from build123d import *

# Parameters (mm, degrees)
EXTRUDE_6_DEPTH           = 20
SKETCH_6_W                = 17.85
SKETCH_6_H                = 4
EXTRUDE_7_DEPTH           = 8
SKETCH_7_W                = 17.85
SKETCH_7_H                = 4
EXTRUDE_8_DEPTH           = 8
SKETCH_10_R               = 1.975
CUT_EXTRUDE_5_DEPTH       = 23.9
SKETCH_9_W                = 11
SKETCH_9_H                = 10.2
CUT_EXTRUDE_7_DEPTH       = 22
SKETCH_12_R               = 3.5
CUT_EXTRUDE_8_DEPTH       = 2.9
CUT_EXTRUDE_9_DEPTH       = 3.2
EXTRUDE_11_DEPTH          = 4
EXTRUDE_START             = -20
EXTRUDE_12_DEPTH          = 20
CUT_EXTRUDE_12_DEPTH      = 10
SKETCH_20_W               = 6
SKETCH_20_H               = 4
CUT_EXTRUDE_13_DEPTH      = 10
REVOLVE_1_ANGLE           = 180
EXTRUDE_13_DEPTH          = 30
SKETCH_38_W               = 28
SKETCH_38_H               = 8
EXTRUDE_14_DEPTH          = 34
SKETCH_37_W               = 8.80839151
SKETCH_37_H               = 35.661760673
CUT_EXTRUDE_15_DEPTH      = 22.758116413
CUT_EXTRUDE_15_DEPTH_BACK = 58.758116413
SKETCH_40_W               = 21.302771057
SKETCH_40_H               = 34
CUT_EXTRUDE_16_DEPTH      = 7
CUT_EXTRUDE_16_DEPTH_BACK = 40.8500001
SKETCH_42_W               = 6
SKETCH_42_H               = 6
CUT_EXTRUDE_17_DEPTH      = 29.0000001
FILLET_1_R                = 5
FILLET_2_R                = 2


with BuildPart() as part:
    # 스케치1 → 보스-돌출6 (new body)
    with BuildSketch(Plane.XY):
        Polygon((-42.18773019, 15.20361991), (-19.28773019, 15.20361991), (-19.28773019, -6.79638009), (3.66226981, -6.79638009), (3.66226981, -77.79638009), (-42.18773019, -77.79638009), (-42.18773019, -73.79638009), (-16.33773019, -73.79638009), (-16.33773019, -26.79638009), (-42.18773019, -26.79638009), align=None)
    extrude(amount=EXTRUDE_6_DEPTH)

    # 스케치6 → 보스-돌출7 (add)
    with BuildSketch(Plane.XY.offset(20)):
        with Locations((-33.26273019, -75.79638009)):
            Rectangle(SKETCH_6_W, SKETCH_6_H)
    extrude(amount=EXTRUDE_7_DEPTH)

    # 스케치7 → 보스-돌출8 (add)
    with BuildSketch(Plane(origin=(0, 0, 0), x_dir=(-1, 0, 0), z_dir=(0, 0, -1))):
        with Locations((33.26273019, -75.79638009)):
            Rectangle(SKETCH_7_W, SKETCH_7_H)
    extrude(amount=EXTRUDE_8_DEPTH)

    # 스케치10 → 컷-돌출5 (cut, through all)
    with BuildSketch(Plane(origin=(-19.28773019, 0, 0), x_dir=(0, 0, -1), z_dir=(1, 0, 0))):
        with Locations((-10, 10.20361991)):
            Circle(SKETCH_10_R)
        with Locations((-10, -0.79638009)):
            Circle(SKETCH_10_R)
    extrude(amount=-CUT_EXTRUDE_5_DEPTH, mode=Mode.SUBTRACT)

    # 스케치9 → 컷-돌출7 (cut)
    with BuildSketch(Plane(origin=(0, 15.20361991, 0), x_dir=(1, 0, 0), z_dir=(0, 1, 0))):
        with Locations((-31.28773019, -10)):
            Rectangle(SKETCH_9_W, SKETCH_9_H)
    extrude(amount=-CUT_EXTRUDE_7_DEPTH, mode=Mode.SUBTRACT)

    # 스케치12 → 컷-돌출8 (cut)
    with BuildSketch(Plane(origin=(-19.28773019, 0, 0), x_dir=(0, 0, -1), z_dir=(1, 0, 0))):
        with Locations((-10, 10.20361991)):
            Circle(SKETCH_12_R)
        with Locations((-10, -0.79638009)):
            Circle(SKETCH_12_R)
    extrude(amount=-CUT_EXTRUDE_8_DEPTH, mode=Mode.SUBTRACT)

    # 스케치13 → 컷-돌출9 (cut)
    with BuildSketch(Plane.ZY.offset(42.18773019)):
        Polygon((10, 14.360541848), (6.4, 12.282080879), (6.4, 8.12515894), (10, 6.046697971), (13.6, 8.12515894), (13.6, 12.282080879), align=None)
        Polygon((10, 3.360541848), (6.4, 1.282080879), (6.4, -2.87484106), (10, -4.953302029), (13.6, -2.87484106), (13.6, 1.282080879), align=None)
    extrude(amount=-CUT_EXTRUDE_9_DEPTH, mode=Mode.SUBTRACT)

    # 스케치16 → 보스-돌출11 (add)
    with BuildSketch(Plane(origin=(0, -73.79638009, 0), x_dir=(1, 0, 0), z_dir=(0, 1, 0))):
        with BuildLine():
            Line((-16.33773019, -20), (-24.33773019, -20))
            Line((-24.33773019, -20), (-24.33773019, -28))
            ThreePointArc((-24.33773019, -28), (-18.680875941, -25.656854249), (-16.33773019, -20))
        make_face()
        with BuildLine():
            Line((-16.33773019, 0), (-24.33773019, 0))
            Line((-24.33773019, 0), (-24.33773019, 8))
            ThreePointArc((-24.33773019, 8), (-18.680875941, 5.656854249), (-16.33773019, 0))
        make_face()
    extrude(amount=-EXTRUDE_11_DEPTH)

    # 스케치17 → 보스-돌출12 (add)
    with BuildSketch(Plane.XY.offset(20).offset(EXTRUDE_START)):
        with BuildLine():
            Line((-22.33773019, -73.79638009), (-16.33773019, -73.79638009))
            Line((-16.33773019, -73.79638009), (-16.33773019, -67.79638009))
            ThreePointArc((-16.33773019, -67.79638009), (-18.095089503, -72.039020778), (-22.33773019, -73.79638009))
        make_face()
    extrude(amount=EXTRUDE_12_DEPTH)

    # 스케치8 → 컷-돌출12 (cut)
    with BuildSketch(Plane.XZ.offset(77.79638009)):
        with BuildLine():
            Line((-42.18773019, 23), (-42.18773019, -3))
            ThreePointArc((-42.18773019, -3), (-29.18773019, 10), (-42.18773019, 23))
        make_face()
    extrude(amount=-CUT_EXTRUDE_12_DEPTH, mode=Mode.SUBTRACT)

    # 스케치20 → 컷-돌출13 (cut)
    with BuildSketch(Plane.XY.offset(28)):
        with Locations((-39.18773019, -75.79638009)):
            Rectangle(SKETCH_20_W, SKETCH_20_H)
    extrude(amount=-CUT_EXTRUDE_13_DEPTH, mode=Mode.SUBTRACT)

    # 스케치32 → 회전1 (revolve)
    with BuildSketch(Plane.ZY.offset(42.18773019)):
        with BuildLine():
            Line((-8, -77.79638009), (-3, -77.79638009))
            ThreePointArc((-3, -77.79638009), (-15.841250436, -90.997978116), (-23.39066063, -107.79638009))
            Line((-23.39066063, -107.79638009), (-29.758116313, -107.79638009))
            ThreePointArc((-29.758116313, -107.79638009), (-21.866282132, -88.884722246), (-8, -73.79638009))
            Line((-8, -73.79638009), (-8, -77.79638009))
        make_face()
    revolve(axis=Axis((-42.18773019, -67.79638009, 10), (0, -1, 0)), revolution_arc=REVOLVE_1_ANGLE)

    # 스케치33 → 보스-돌출13 (add)
    with BuildSketch(Plane.XZ.offset(77.79638009)):
        with BuildLine():
            Line((3.66226981, 20), (3.66226981, 0))
            Line((3.66226981, 0), (-16.33773019, 0))
            ThreePointArc((-16.33773019, 0), (-18.680875941, -5.656854249), (-24.33773019, -8))
            Line((-24.33773019, -8), (-28.366850202, -8))
            ThreePointArc((-28.366850202, -8), (-19.493750292, 10), (-28.366850202, 28))
            Line((-28.366850202, 28), (-24.33773019, 28))
            ThreePointArc((-24.33773019, 28), (-18.680875941, 25.656854249), (-16.33773019, 20))
            Line((-16.33773019, 20), (3.66226981, 20))
        make_face()
    extrude(amount=EXTRUDE_13_DEPTH)

    # 스케치38 → 보스-돌출14 (add)
    with BuildSketch(Plane(origin=(0, -73.79638009, 0), x_dir=(1, 0, 0), z_dir=(0, 1, 0))):
        with Locations((-10.33773019, 4)):
            Rectangle(SKETCH_38_W, SKETCH_38_H)
        with Locations((-10.33773019, -24)):
            Rectangle(SKETCH_38_W, SKETCH_38_H)
    extrude(amount=-EXTRUDE_14_DEPTH)

    # 스케치39 → 컷-회전1 (revolve, cut)
    with BuildSketch(Plane.ZY.offset(42.18773019)):
        with BuildLine():
            Line((10, -107.79638009), (-23.39066063, -107.79638009))
            ThreePointArc((-23.39066063, -107.79638009), (-15.841250436, -90.997978116), (-3, -77.79638009))
            Line((-3, -77.79638009), (10, -77.79638009))
            Line((10, -77.79638009), (10, -107.79638009))
        make_face()
    revolve(axis=Axis((-42.18773019, -107.79638009, 10), (0, 1, 0)), mode=Mode.SUBTRACT)

    # 스케치37 → 컷-돌출15 (cut, two sides)
    with BuildSketch(Plane.XY.offset(28)) as cut_extrude_15_sk:
        with Locations((-40.591925945, -91.627260427)):
            Rectangle(SKETCH_37_W, SKETCH_37_H)
    extrude(amount=CUT_EXTRUDE_15_DEPTH, mode=Mode.SUBTRACT)
    extrude(cut_extrude_15_sk.sketch, amount=-CUT_EXTRUDE_15_DEPTH_BACK, mode=Mode.SUBTRACT)

    # 스케치40 → 컷-돌출16 (cut, two sides)
    with BuildSketch(Plane.ZY.offset(36.18773019)) as cut_extrude_16_sk:
        with Locations((-18.651385529, -90.79638009)):
            Rectangle(SKETCH_40_W, SKETCH_40_H)
        with Locations((38.651385529, -90.79638009)):
            Rectangle(SKETCH_40_W, SKETCH_40_H)
    extrude(amount=CUT_EXTRUDE_16_DEPTH, mode=Mode.SUBTRACT)
    extrude(cut_extrude_16_sk.sketch, amount=-CUT_EXTRUDE_16_DEPTH_BACK, mode=Mode.SUBTRACT)

    # 스케치42 → 컷-돌출17 (cut, through all)
    with BuildSketch(Plane.XY.offset(20)):
        with Locations((-19.33773019, -70.79638009)):
            Rectangle(SKETCH_42_W, SKETCH_42_H)
    extrude(amount=-CUT_EXTRUDE_17_DEPTH, mode=Mode.SUBTRACT)

    # 필렛1
    fillet_1_edges = [part.edges().sort_by_distance(p)[0] for p in [
        (-6.33773019, -73.79638009, 20),
        (-6.33773019, -73.79638009, 0),
        (-16.33773019, -73.79638009, 10),
    ]]
    fillet(fillet_1_edges, radius=FILLET_1_R)

    # 필렛2
    fillet_2_edges = [part.edges().sort_by_distance(p)[0] for p in [
        (-36.18773019, -75.79638009, 21.532562595),
        (-36.18773019, -75.79638009, -1.532562595),
    ]]
    fillet(fillet_2_edges, radius=FILLET_2_R)


solid = part.part
Here's how the part is built. I have some questions about the finished solid (model axes, mm). A direction names the side the tool comes from. Coordinates: 2 decimals unless noted, no trailing zeros. Order: outer loops, then holes, each group sorted by start corner. A loop starts at its lowest first (then second) coordinate and runs counter-clockwise, first axis right, second up. Notation, with made-up numbers: M 76,9.25 L 135,9.25 A26 ccw 135,25.25 Z; hole C 6,89.5 d11. An arc over 180 degrees is marked long. Answer as CSV lines item,"result".
Item 1: On a 3-axis mill with a long thin cutter (end or side, diameter ignored), from which of +Z, -Z, +X, -X, +Y, -Y can I reach the whole of each face in a straight line? I mean faces 1 (the face through (-20, -26, 20)), 2 (the face through (-20.717, 13.674, 10.456)), 3 (the face through (-25.788, 4, 10)), 4 (the face through (-25, -73.796, 10)). Say none if no direction works.
Results found:
face 1,"+Z, +X, -X, +Y"
face 2,"+X"
face 3,"+Y"
face 4,"-X"
Item 2: We'd pull the mould along Y, two halves only. Please class faces 5 (the face through (-23.963, -1.553, 8.176)), 6 (the face through (-31, 4, 15.1)): +Y half, -Y half, draft (parallel to the pull), parting line (faces both ways), or undercut.
Results found:
face 5,"undercut"
face 6,"draft"
Item 3: If I drill on line 1 (Y direction, x = -37, z = 10); line 2 (Y direction, x = -23, z = 10); line 3 (Y direction, x = -20, z = 10), over which ranges is the centre line in solid material (lowest first)?
Results found:
line 1,"-26.8 to -2.77, 1.18 to 8.23, 12.18 to 15.2"
line 2,"-83.02 to -73.8, -26.8 to -2.77, 1.18 to 8.23, 12.18 to 15.2"
line 3,"-86.23 to -73.61, -26.8 to -4.3, 2.7 to 6.7, 13.7 to 15.2"
Item 4: Imagine slicing it at B-B on x = -33.5. Give the number of separate pieces and of enclosed holes in the cut face, plus the area to 3 significant figures.
Results found:
separate pieces,"3"
enclosed holes,"0"
area,"728 mm2"
Item 5: Imagine slicing it at A-A on y = -35.5. Write out the boundary of the cut face in (x, z).
Results found:
outline,"M -16.34,0 L 3.66,0 L 3.66,20 L -16.34,20 Z"
Item 6: For pin 1 (12 mm diameter, centred on x = -11.5, y = -32, fed in from -Z); pin 2 (9 mm diameter, centred on x = -30, y = 7, fed in from +Z); pin 3 (2 mm diameter, centred on y = -2.5, z = 9, fed in from +X), each with a flat end and sliding along its axis, tell me the tip position at first contact or that it passes through.
Results found:
pin 1,"z = 0"
pin 2,"z = 20"
pin 3,"x = -22.19"
Item 7: Imagine slicing it at C-C on y = -10.5. Write out the boundary of the cut face in (x, z), plus the area to 3 significant figures.
Results found:
outline,"M -42.19,0 L 3.66,0 L 3.66,20 L -42.19,20 Z"
area,"917 mm2"
